from build123d import *

# Parameters (mm, degrees)
F0_W     = 12
F0_H     = 2
F2_R     = 1
F3_R     = 5.5
F4_DEPTH = 0.5
F5_R     = 4.025
F6_DEPTH = 3
F7_R     = 1


with BuildPart() as f1:
    # F0 (on Front) → F1 (revolve)
    with BuildSketch(Plane.XZ):
        with Locations((6, 1)):
            Rectangle(F0_W, F0_H)
    revolve(axis=Axis((0, 0, 1), (0, 0, 1)))

    # F2
    f2_edges = [f1.edges().sort_by_distance(p)[0] for p in [
        (-12, 0, 2),
    ]]
    fillet(f2_edges, radius=F2_R)

    # F3 (on face) → F4 (join)
    with BuildSketch(Plane(origin=(0, 0, 0), x_dir=(1, 0, 0), z_dir=(0, 0, -1))):
        Circle(F3_R)
    extrude(amount=F4_DEPTH)

    # F5 (on face) → F6 (join)
    with BuildSketch(Plane(origin=(0, 0, -0.5), x_dir=(1, 0, 0), z_dir=(0, 0, -1))):
        Circle(F5_R)
    extrude(amount=F6_DEPTH)

    # F7
    f7_edges = [f1.edges().sort_by_distance(p)[0] for p in [
        (-4.025, 0, -3.5),
    ]]
    fillet(f7_edges, radius=F7_R)


solid = f1.part
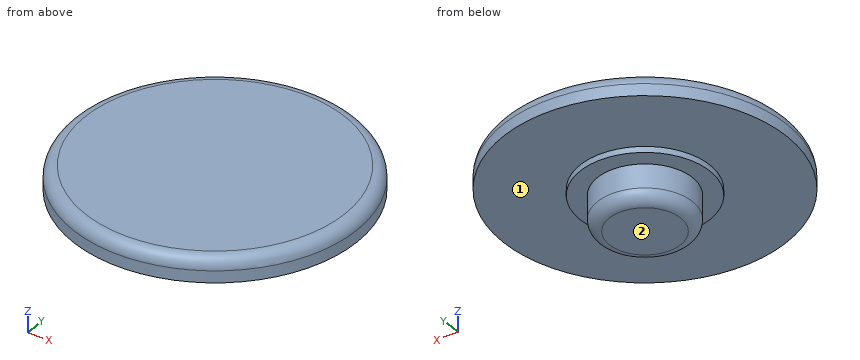
Can you work these out from the model? Positions are in its coordinate system, mm. Face numbers are marked on the shaded views. A direction names the side the tool comes from. Coordinates: 2 decimals unless noted, no trailing zeros. Order: outer loops, then holes, each group sorted by start corner. A loop starts at its lowest first (then second) coordinate and runs counter-clockwise, first axis right, second up. Notation, with made-up numbers: (-4.5, 10.5) - (45.5, 10.5) arc R17 ccw to (45.5, 29.5) - close; hole circle Ø4 at (31.5, 26.25). An arc over 180 degrees is marked (long way). Answer as a JSON object with one key per item and string values. Group by question number.
Q1. Imagine slicing it at A-A (y = 0). Please give me the cut outline in (x, z) (3 decimals), and give its area (3 significant figures).
Q2. Will this pin go through, and if not, where does the flat tip stop? P1, Ø3, axis at y = -6, z = -3, coming from the -X side.
Q3. Imagine slicing it at C-C (z = -3). Please give me the cut outline in (x, y), and give its area (3 significant figures).
Q4. On a 3-axis mill with a long thin cutter (end or side, diameter ignored), from which of +Z, -Z, +X, -X, +Y, -Y can I reach the whole of each face in a straight line? I mean the marked faces 1 and 2. Say none if no direction works.
Q5. I need wall thicknesses on line 1 (Y direction, x = 0, z = -1.55) (3 decimals); line 2 (Z direction, x = -0.5, y = 11); line 3 (Z direction, x = 1.5, y = 4.75). Which ranges of each line are inside material? Lowest first, please. Write a range as from..to.
Determined:
{
 "1": {"outline": "(-12, 0) - (-5.5, 0) - (-5.5, -0.5) - (-4.025, -0.5) - (-4.025, -2.5) arc R1 ccw to (-3.025, -3.5) - (3.025, -3.5) arc R1 ccw to (4.025, -2.5) - (4.025, -0.5) - (5.5, -0.5) - (5.5, 0) - (12, 0) - (12, 1) arc R1 ccw to (11, 2) - (-11, 2) arc R1 ccw to (-12, 1) - close", "area": "76.8 mm2"},
 "2": {"P1": "passes through"},
 "3": {"outline": "circle Ø7.78 at (0, 0)", "area": "47.6 mm2"},
 "4": {"face 1": "-Z", "face 2": "-Z, +X, -X, +Y, -Y"},
 "5": {"line 1": "y = -4.025..4.025", "line 2": "z = 0..2", "line 3": "z = -0.5..2"}
}
